Read the model definition and answer for the solid it produces. Units are mm, in the model's axes. A direction names the side the tool comes from. Give positions to 0.01 mm unless a question says otherwise; leave off trailing zeros. Loops run counter-clockwise (first coordinate to the right, second up) from the corner with the lowest first, then second, coordinate; pieces in that order, holes last. Notation, with made-up numbers: (15, 31.25) - (51, 31.25) arc R26 cw to (51, 68.25) - close; hole circle Ø5 at (57.5, 7). An arc over 180 degrees is marked (long way). Use a Markdown table: item, result. Add a question column.
Item 1: A cutting plane is placed at D-D (y = 35.5). Determine the outline of the cut face in (x, z), plus the area to 3 significant figures.
Item 2: A cutting plane is placed at A-A (y = 120.5). Give the number of separate pieces and of enclosed holes in the cut face, plus the area to 3 significant figures.
Item 3: Consider probe 1 along Z at (x, y) = (142.5, 96.5); probe 2 along X at (y, z) = (102.5, 9); probe 3 along X at (y, z) = (112, 62). Determine where each line is inside the solid, lowest interval first. Write a range as [from, to].
Item 4: Each of these flat-tipped pins is pushed along its axis until it touches: P1, Ø1.5, axis at y = 111, z = 19, coming from the -X side; P2, Ø10, axis at x = 249.5, z = 0, coming from the +Y side. Where does it stop, or does it pass through?
Item 5: A cutting plane is placed at C-C (z = 46). Determine the outline of the cut face in (x, y).
Item 6: For a pull along X with two mould halves and no side action, classify faces 1 (the face through (-250, 110, 0)), 2 (the face through (-3, 81, -55)) as +X half, -X half, draft (parallel to the pull), parting line (faces both ways), or undercut.
Item 7: Which of the six approach directions +Z, -Z, +X, -X, +Y, -Y give full straight-line access (tool end or side, diameter ignored) to faces 3 (the face through (0, 130, -60)), 4 (the face through (250, 125, -20)), 5 (the face through (240, 81, 1)), 6 (the face through (15, 120, 65)), 7 (the face through (-4, 56, -75))?
from build123d import *

# Parameters (mm, degrees)
SKETCH_1_W           = 520
SKETCH_1_H           = 150
EXTRUDE_1_DEPTH      = 140
SKETCH_2_W           = 480
SKETCH_2_H           = 110
CUT_EXTRUDE_1_DEPTH  = 120
SKETCH_11_W          = 40
SKETCH_11_H          = 30
CUT_EXTRUDE_3_DEPTH  = 544.714079273
SKETCH_13_W          = 520
SKETCH_13_H          = 150
EXTRUDE_6_DEPTH      = 30
SKETCH_18_W          = 30
SKETCH_18_H          = 15.352958973
CUT_EXTRUDE_8_DEPTH  = 30
FILLET_1_R           = 10
SKETCH_21_W          = 30
SKETCH_21_H          = 19.875616275
CUT_EXTRUDE_9_DEPTH  = 30
SKETCH_22_W          = 30
SKETCH_22_H          = 19.88
CUT_EXTRUDE_10_DEPTH = 30
SKETCH_25_W          = 30
SKETCH_25_H          = 19.88
CUT_EXTRUDE_12_DEPTH = 30


with BuildPart() as part:
    # 草圖1 → 填料-伸長1 (new body)
    with BuildSketch(Plane(origin=(0, 0, 0), x_dir=(1, 0, 0), z_dir=(0, 1, 0))):
        Rectangle(SKETCH_1_W, SKETCH_1_H)
    extrude(amount=EXTRUDE_1_DEPTH)

    # 草圖2 → 除料-伸長1 (cut)
    with BuildSketch(Plane(origin=(0, 140, 0), x_dir=(1, 0, 0), z_dir=(0, 1, 0))):
        Rectangle(SKETCH_2_W, SKETCH_2_H)
    extrude(amount=-CUT_EXTRUDE_1_DEPTH, mode=Mode.SUBTRACT)

    # 草圖11 → 除料-伸長3 (cut, through all)
    with BuildSketch(Plane.ZY.offset(260)):
        with Locations((0, 125)):
            Rectangle(SKETCH_11_W, SKETCH_11_H)
    extrude(amount=-CUT_EXTRUDE_3_DEPTH, mode=Mode.SUBTRACT)

    # 草圖13 → 填料-伸長6 (add)
    with BuildSketch(Plane.XZ):
        Rectangle(SKETCH_13_W, SKETCH_13_H)
    extrude(amount=EXTRUDE_6_DEPTH)

    # 草圖18 → 除料-伸長8 (cut)
    with BuildSketch(Plane(origin=(0, 0, -75), x_dir=(-1, 0, 0), z_dir=(0, 0, -1))):
        with Locations((0, 122.323520514)):
            Rectangle(SKETCH_18_W, SKETCH_18_H)
    extrude(amount=-CUT_EXTRUDE_8_DEPTH, mode=Mode.SUBTRACT)

    # 圓角1
    fillet_1_edges = [part.edges().sort_by_distance(p)[0] for p in [
        (0, 130, -75),
    ]]
    fillet(fillet_1_edges, radius=FILLET_1_R - 0.0001)  # a hair under: the kernel refuses the full size

    # 草圖21 → 除料-伸長9 (cut)
    with BuildSketch(Plane.XY.offset(75)):
        with Locations((-195, 120.062191863)):
            Rectangle(SKETCH_21_W, SKETCH_21_H)
    extrude(amount=-CUT_EXTRUDE_9_DEPTH, mode=Mode.SUBTRACT)

    # 草圖22 → 除料-伸長10 (cut)
    with BuildSketch(Plane.XY.offset(75)):
        with Locations((0, 120.06)):
            Rectangle(SKETCH_22_W, SKETCH_22_H)
    extrude(amount=-CUT_EXTRUDE_10_DEPTH, mode=Mode.SUBTRACT)

    # 草圖25 → 除料-伸長12 (cut)
    with BuildSketch(Plane.XY.offset(75)):
        with Locations((205.891066665, 120.06)):
            Rectangle(SKETCH_25_W, SKETCH_25_H)
    extrude(amount=-CUT_EXTRUDE_12_DEPTH, mode=Mode.SUBTRACT)


solid = part.part
Geometry says:
| question | item | result |
|---|---|---|
| 1 | outline | (-260, -75) - (260, -75) - (260, 75) - (-260, 75) - close; hole (-240, -55) - (240, -55) - (240, 55) - (-240, 55) - close |
| 1 | area | 25,200 mm² |
| 2 | separate pieces | 6 |
| 2 | enclosed holes | 0 |
| 2 | area | 21,200 mm² |
| 3 | probe 1 | [-75, -55], [55, 75] |
| 3 | probe 2 | [-260, -240], [240, 260] |
| 3 | probe 3 | [-260, -210], [-180, -15], [15, 190.89], [220.89, 260] |
| 4 | P1 | through |
| 4 | P2 | y = 110 |
| 5 | outline | (-260, -30) - (260, -30) - (260, 140) - (240, 140) - (240, 20) - (-240, 20) - (-240, 140) - (-260, 140) - close |
| 6 | face 1 | draft |
| 6 | face 2 | undercut |
| 7 | face 3 | +Z, -Z |
| 7 | face 4 | +X, -X, +Y |
| 7 | face 5 | +Y |
| 7 | face 6 | +Z |
| 7 | face 7 | -Z, +X, -X, +Y, -Y |
